Part print with two shaded views. Sizes in mm from the minimum x, y, z corner. Give positions to 0.01 mm unless a question says otherwise; leave off trailing zeros. Order: outer loops, then holes, each group sorted by start corner. A loop starts at its lowest first (then second) coordinate and runs counter-clockwise, first axis right, second up. Notation, with made-up numbers: (70, -39) -> (110, -39) arc R25 ccw to (110, -18) -> close; hole circle Ø9 at (0.5, -20). An arc over 180 degrees is marked (long way). Write item = value, one per line. Start each with the question number.
Item 1: Flat gauge pin, fed straight in: P1, Ø3, axis at x = 5.1, z = 177.5, coming from the -Y side. Where does the tip first touch, or does it go through?
Item 2: Drill centre lines: line 1 along X through (y, z) = (2.35, 22.5); line 2 along X through (y, z) = (3.3, 177); line 3 along X through (y, z) = (2.75, 32). Where is each one in solid material? Low to high.
Item 3: Band-saw the part on A-A on x = 210. Write the cut outline in (y, z), plus the area to 3 significant figures.
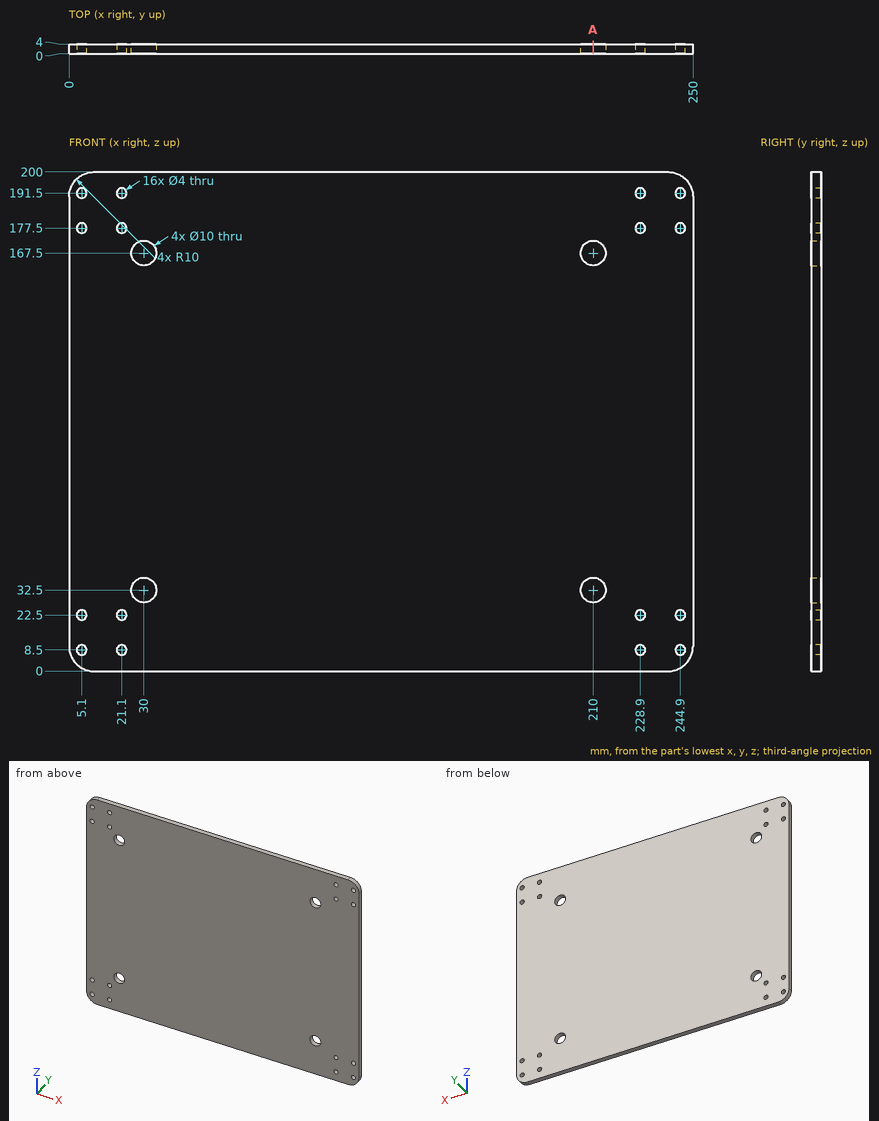
Values found:
q1.P1 = through
q2.line_1 = 0 to 3.1, 7.1 to 19.1, 23.1 to 226.9, 230.9 to 242.9, 246.9 to 250
q2.line_2 = 0 to 3.16, 7.04 to 19.16, 23.04 to 226.96, 230.84 to 242.96, 246.84 to 250
q2.line_3 = 0 to 25.03, 34.97 to 205.03, 214.97 to 250
q3.outline = (0, 0) -> (4, 0) -> (4, 27.5) -> (0, 27.5) -> close; (0, 37.5) -> (4, 37.5) -> (4, 162.5) -> (0, 162.5) -> close; (0, 172.5) -> (4, 172.5) -> (4, 200) -> (0, 200) -> close
q3.area = 720 mm^2
